Could you check a few things on this model? Use its own coordinates, in mm. Coordinates: 2 decimals unless noted, no trailing zeros. Loops run counter-clockwise (first coordinate to the right, second up) from the corner with the lowest first, then second, coordinate; pieces in that order, holes last.
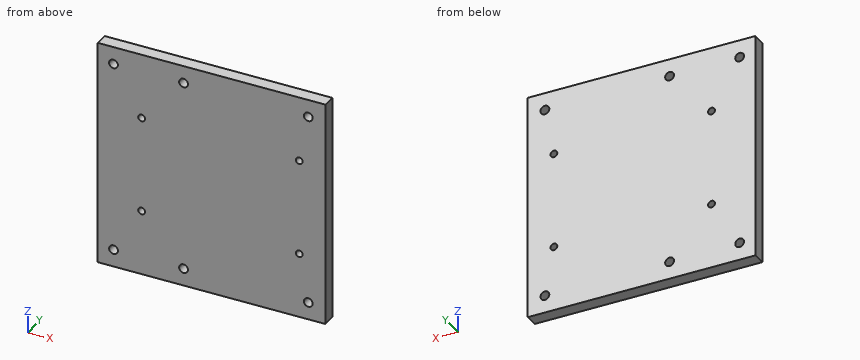
Autodesk Inventor part; units mm, degrees
ref_plane "YZ Plane" through (0, 0, 0) normal (1, 0, 0) x (0, 1, 0)
ref_plane "XZ Plane" through (0, 0, 0) normal (0, 1, 0) x (-1, 0, 0)
ref_plane "XY Plane" through (0, 0, 0) normal (0, 0, 1) x (1, 0, 0)
sketch "Sketch2" plane through (0, 0, 0) normal (0, 1, 0) x (-1, 0, 0)
  line L0 (82.55, 82.55) -> (-82.55, 82.55)
  line L1 (-82.55, 82.55) -> (-82.55, -82.55)
  line L2 (-82.55, -82.55) -> (82.55, -82.55)
  line L3 (82.55, -82.55) -> (82.55, 82.55)
  point P0 (0, 0)
  point P1 (82.55, 0)
  point P2 (0, -82.55)
  dimension "d0" = 165.1
  dimension "d1" = 165.1
extrude "Extrusion1" add sketch "Sketch2" along normal blind 9.525
sketch "Sketch3" plane through (0, 9.525, 0) normal (0, 1, 0) x (1, 0, 0)
  line L0 (-82.55, 82.55) -> (-82.55, -82.55)
  line L1 (82.55, 82.55) -> (-82.55, 82.55)
  line L2 (115.57, 0) -> (-115.57, 0)
  point P0 (0, 0)
  point P1 (-71.12, 69.85)
  point P2 (-20.32, 69.85)
  point P3 (70.104, 69.85)
  point P4 (-71.12, -69.85)
  point P5 (-20.32, -69.85)
  point P6 (70.104, -69.85)
  dimension "d4" = 11.43
  dimension "d5" = 50.8
  dimension "d6" = 90.424
  dimension "d7" = 12.7
hole "Hole1" at (-71.12, 9.525, -69.85) at (-20.32, 9.525, -69.85) at (70.104, 9.525, -69.85) at (-71.12, 9.525, 69.85) at (-20.32, 9.525, 69.85) at (70.104, 9.525, 69.85) direction (0, -1, 0) diameter 6.4008 end through all
sketch "Sketch4" plane through (0, 9.525, 0) normal (0, 1, 0) x (1, 0, 0)
  circle A0 centre (-20.32, -69.85) radius 3.2004
  circle A1 centre (70.104, 69.85) radius 3.2004
  circle A2 centre (-71.12, 69.85) radius 3.2004
  circle A3 centre (-20.32, 69.85) radius 3.2004
  circle A4 centre (-71.12, -69.85) radius 3.2004
  circle A5 centre (70.104, -69.85) radius 3.2004
  line L0 (-82.55, -82.55) -> (82.55, -82.55)
  line L1 (82.55, -82.55) -> (82.55, 82.55)
  line L2 (82.55, 82.55) -> (-82.55, 82.55)
  line L3 (-82.55, 82.55) -> (-82.55, -82.55)
  line L4 (-115.57, 0) -> (115.57, 0)
  point P0 (0, 0)
  point P1 (-50.7238, 35.0012)
  point P2 (63.5762, 35.0012)
  point P3 (-50.7238, -35.0012)
  point P4 (63.5762, -35.0012)
  dimension "d15" = 31.8262
  dimension "d16" = 114.3
  dimension "d17" = 47.5488
hole "Hole2" at (-50.7238, 9.525, -35.0012) at (63.5762, 9.525, -35.0012) at (-50.7238, 9.525, 35.0012) at (63.5762, 9.525, 35.0012) direction (0, -1, 0) diameter 4.9784 end through all
properties part number "Motor Shim"
(1) I need wall thicknesses on probe 1 along Z at (x, y) = (-71.12, 5); probe 2 along Z at (x, y) = (-50.5, 6); probe 3 along X at (y, z) = (6, 69.85). Which ranges of each line are inside material? Lowest first, please.
Answers:
probe 1: z = -82.55 to -73.05, -66.65 to 66.65, 73.05 to 82.55
probe 2: z = -82.55 to -37.48, -32.52 to 32.52, 37.48 to 82.55
probe 3: x = -82.55 to -74.32, -67.92 to -23.52, -17.12 to 66.9, 73.3 to 82.55
(2) For pin 1 (4 mm diameter, centred on x = -50.72, z = -35, fed in from -Y); pin 2 (5.5 mm diameter, centred on x = -50.72, z = 35, fed in from -Y), each with a flat end and sliding along its axis, tell me the tip position at first contact or that it passes through.
Answers:
pin 1: passes through
pin 2: stops at y = 0
(3) Imagine slicing it at B-B, the plane z = 69.85. Write out the boundary of the cut face in (x, y) (3 decimals), and give its area (3 significant figures).
Answers:
outline: (-82.55, 0) - (-74.32, 0) - (-74.32, 9.525) - (-82.55, 9.525) - close; (-67.92, 0) - (-23.52, 0) - (-23.52, 9.525) - (-67.92, 9.525) - close; (-17.12, 0) - (66.904, 0) - (66.904, 9.525) - (-17.12, 9.525) - close; (73.304, 0) - (82.55, 0) - (82.55, 9.525) - (73.304, 9.525) - close
area: 1,390 mm2
(4) Imagine slicing it at A-A, the plane x = -20.32. Write out the boundary of the cut face in (y, z) (3 decimals), and give its area (3 significant figures).
Answers:
outline: (0, -82.55) - (9.525, -82.55) - (9.525, -73.05) - (0, -73.05) - close; (0, -66.65) - (9.525, -66.65) - (9.525, 66.65) - (0, 66.65) - close; (0, 73.05) - (9.525, 73.05) - (9.525, 82.55) - (0, 82.55) - close
area: 1,450 mm2
